Could you check a few things on this drawing? It's one solid part, dimensions in mm from its lowest x, y, z. A direction names the side the tool comes from. Round coordinates to 2 decimals unless told otherwise and drop trailing zeros. Loops run counter-clockwise (first coordinate to the right, second up) from the corner with the lowest first, then second, coordinate; pieces in that order, holes last. Notation, with made-up numbers: (55, -4) -> (77, -4) arc R19 cw to (77, 3) -> close; hole circle Ø10 at (-32.75, -25). An arc over 180 degrees is marked (long way). Use CSV: the item, a comma, the result in double quotes. Start each with the question number.
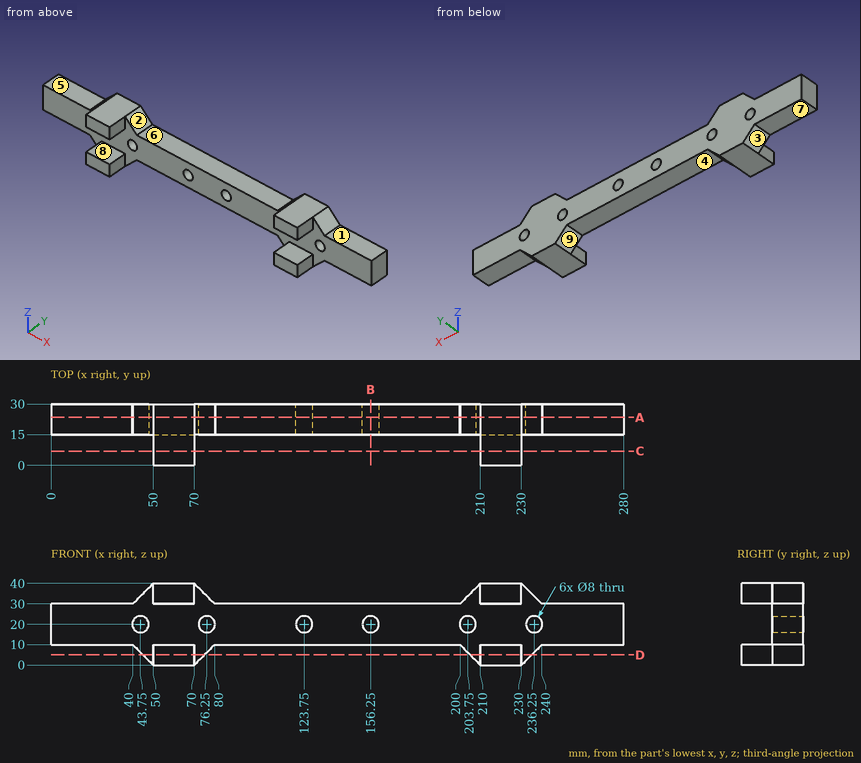
Q1. I want a section at B-B, the plane x = 156.25. List the corners of the cut face in (y, z) for me.
Q2. I want a section at A-A, the plane y = 23.5. Count the separate pieces of the cut face and the enclosed holes in it, then the cut area to 3 significant figures.
Q3. Will these pins go through, and if not, where does the flat tip stop? pin 1 Ø7.5 at (x, y) = (261.5, 25.5) entering from +Z; pin 2 Ø3 at (y, z) = (15.5, 36.5) entering from -X; pin 3 Ø5 at (x, z) = (76.25, 20) entering from -Y; pin 4 Ø12 at (x, z) = (162.5, 20) entering from -Y.
Q4. For the marked faces 5, 6, 7, 8 and 9, which set-ups out of +Z, -Z, +X, -X, +Y, -Y let a thin tool reach every point of the face, with its end or its side?
Q5. I need wall thicknesses on line 1 along X through (y, z) = (8, 3.5); line 2 along Z through (x, y) = (57.5, 7.5); line 3 along Y through (x, z) = (139, 19). Which ranges of each line are inside material? Lowest first, please.
Q6. I want a section at C-C, the plane y = 7. List the corners of the cut face in (x, z) for me, then the cut area to 3 significant figures.
Q7. I want a section at D-D, the plane z = 5. List the corners of the cut face in (x, y) for me.
Q8. If we mould it in two halves opening along X, with no side actions, what happens to the marked faces 1, 2, 3 and 4? For each: pulls with the +X half, pulls with the -X half, needs draft (parallel to the pull), parting line crosses it, or undercut.
Values found:
1,outline,"(15, 10) -> (30, 10) -> (30, 16) -> (15, 16) -> close; (15, 24) -> (30, 24) -> (30, 30) -> (15, 30) -> close"
2,separate pieces,"1"
2,enclosed holes,"6"
2,area,"6,500 mm2"
3,pin 1,"z = 30"
3,pin 2,"x = 45"
3,pin 3,"through"
3,pin 4,"y = 15"
4,face 5,"+Z, -X, +Y, -Y"
4,face 6,"+Z, +Y, -Y"
4,face 7,"-Z, -X, +Y, -Y"
4,face 8,"+X, -X, -Y"
4,face 9,"-Z, +Y, -Y"
5,line 1,"50 to 70, 210 to 230"
5,line 2,"0 to 10, 30 to 40"
5,line 3,"15 to 30"
6,outline,"(50, 0) -> (70, 0) -> (70, 10) -> (50, 10) -> close; (50, 30) -> (70, 30) -> (70, 40) -> (50, 40) -> close; (210, 0) -> (230, 0) -> (230, 10) -> (210, 10) -> close; (210, 30) -> (230, 30) -> (230, 40) -> (210, 40) -> close"
6,area,"800 mm2"
7,outline,"(45, 15) -> (50, 15) -> (50, 0) -> (70, 0) -> (70, 15) -> (75, 15) -> (75, 30) -> (45, 30) -> close; (205, 15) -> (210, 15) -> (210, 0) -> (230, 0) -> (230, 15) -> (235, 15) -> (235, 30) -> (205, 30) -> close"
8,face 1,"needs draft"
8,face 2,"undercut"
8,face 3,"pulls with the -X half"
8,face 4,"undercut"
